The model under review builds one solid part; all positions refer to its coordinate system, in mm. A direction names the side the tool comes from. Give positions to 0.01 mm unless a question says otherwise; leave off trailing zeros. Order: outer loops, then holes, each group sorted by start corner. A loop starts at its lowest first (then second) coordinate and runs counter-clockwise, first axis right, second up. Notation, with made-up numbers: (-24, 7.5) - (31, 7.5) arc R16 cw to (31, 38.5) - close; hole circle Ø9 at (-19, 4). An arc over 180 degrees is marked (long way). Use CSV: the item, a comma, the result in double quotes. Start each with the question number.
```python
from build123d import *

# Parameters (mm, degrees)
BOSS_EXTRUDE1_DEPTH                             = 53.975
SKETCH2_W                                       = 6.858
SKETCH2_H                                       = 3.429
CUT_EXTRUDE1_DEPTH                              = 55.91468839
SKETCH4_W                                       = 6.858
SKETCH4_H                                       = 3.429
CUT_EXTRUDE2_DEPTH                              = 55.91468839
F_3_CLEARANCE_HOLE1_D                           = 2.7686
CBORE_FOR_10_BUTTON_HEAD_CAP_SCREW1_D           = 5.1054
CBORE_FOR_10_BUTTON_HEAD_CAP_SCREW1_CBORE_D     = 9.92124
CBORE_FOR_10_BUTTON_HEAD_CAP_SCREW1_CBORE_DEPTH = 3.2004
FILLET1_R                                       = 1.27
FILLET3_R                                       = 1.27
FILLET5_R                                       = 1.27


with BuildPart() as part:
    # Sketch1 → Boss-Extrude1 (new body)
    with BuildSketch(Plane.XY.offset(23.6855)):
        Polygon((3.302, 6.35), (-4.064, 6.35), (-4.064, -6.35), (3.302, -6.35), (7.874, -2.54), (7.874, 2.54), align=None)
    extrude(amount=-BOSS_EXTRUDE1_DEPTH)

    # Sketch2 → Cut-Extrude1 (cut, through all)
    with BuildSketch(Plane.XY.offset(23.6855)):
        with Locations((-0.635, 4.6355)):
            Rectangle(SKETCH2_W, SKETCH2_H)
    extrude(amount=-CUT_EXTRUDE1_DEPTH, mode=Mode.SUBTRACT)

    # Sketch4 → Cut-Extrude2 (cut, through all)
    with BuildSketch(Plane.XY.offset(23.6855)):
        with Locations((-0.635, -4.6355)):
            Rectangle(SKETCH4_W, SKETCH4_H)
    extrude(amount=-CUT_EXTRUDE2_DEPTH, mode=Mode.SUBTRACT)

    # #3 Clearance Hole1 (through all)
    with Locations(Plane.ZY.offset(4.064)):
        with Locations((12.7, 0), (-12.7, 0)):
            Hole(F_3_CLEARANCE_HOLE1_D / 2)

    # CBORE for #10 Button Head Cap Screw1 (through all)
    with Locations(Plane(origin=(7.874, 0, 0), x_dir=(0, 0, -1), z_dir=(1, 0, 0))):
        with Locations((-12.7, 0), (12.7, 0)):
            CounterBoreHole(CBORE_FOR_10_BUTTON_HEAD_CAP_SCREW1_D / 2, CBORE_FOR_10_BUTTON_HEAD_CAP_SCREW1_CBORE_D / 2, CBORE_FOR_10_BUTTON_HEAD_CAP_SCREW1_CBORE_DEPTH)

    # Fillet1
    fillet1_edges = [part.edges().sort_by_distance(p)[0] for p in [
        (7.874, -2.54, 20.323251747),
        (7.874, -2.54, -23.625251747),
        (7.874, -2.54, 0),
        (7.874, 2.54, 20.323251747),
        (7.874, 2.54, 0),
        (7.874, 2.54, -23.625251747),
    ]]
    fillet(fillet1_edges, radius=FILLET1_R)

    # Fillet3
    # the kernel refuses this fillet: 1.27 mm, written as the material it takes off along each edge
    with BuildSketch(Plane(origin=(0.862897437, -8.382585469, -30.2895), x_dir=(0, 0, 1), z_dir=(0.7682212795973759, 0.6401843996644799, 0)), Plane(origin=(7.417034188, 2.920804844, -30.2895), x_dir=(0, 0, 1), z_dir=(-0.7682212795973759, 0.6401843996644799, 0))) as fillet3_piece_1:
        with BuildLine():
            CenterArc((FILLET3_R, -FILLET3_R), FILLET3_R, 90, 90)
            Line((0, -FILLET3_R), (0, 0))
            Line((0, 0), (FILLET3_R, 0))
        make_face()
    extrude(amount=8.531574072, mode=Mode.SUBTRACT)
    with BuildSketch(Plane(origin=(6.604, -1.945163819, -30.2895), x_dir=(0.6401843996644796, -0.7682212795973762, 0), z_dir=(-0.7682212795973762, -0.6401843996644796, 0))) as fillet3_piece_2:
        with BuildLine():
            CenterArc((1.27 - FILLET3_R, FILLET3_R), FILLET3_R, 270, 90)
            Line((1.27, FILLET3_R), (1.27, 0))
            Line((1.27, 0), (1.27 - FILLET3_R, 0))
        make_face()
    revolve(axis=Axis((6.604, -1.945163819, -30.2895), (0, 0, 1)), revolution_arc=50.194428908, mode=Mode.SUBTRACT)
    with BuildSketch(Plane(origin=(6.604, 1.945163819, -30.2895), x_dir=(0.6401843996644799, 0.7682212795973757, 0), z_dir=(-0.7682212795973757, 0.6401843996644799, 0))) as fillet3_piece_3:
        with BuildLine():
            CenterArc((1.27 - FILLET3_R, -FILLET3_R), FILLET3_R, 0, 90)
            Line((1.27, -FILLET3_R), (1.27, 0))
            Line((1.27, 0), (1.27 - FILLET3_R, 0))
        make_face()
    revolve(axis=Axis((6.604, 1.945163819, -30.2895), (0, 0, -1)), revolution_arc=50.194428908, mode=Mode.SUBTRACT)
    with BuildSketch(Plane(origin=(2.794, -2.921, -30.2895), x_dir=(0, 0, 1), z_dir=(-1, 0, 0)), Plane(origin=(-7.239, 2.921, -30.2895), x_dir=(0, 0, 1), z_dir=(1, 0, 0))) as fillet3_piece_4:
        with BuildLine():
            CenterArc((FILLET3_R, FILLET3_R), FILLET3_R, 180, 90)
            Line((0, FILLET3_R), (0, 0))
            Line((0, 0), (FILLET3_R, 0))
        make_face()
    extrude(amount=10.033, mode=Mode.SUBTRACT)
    with BuildSketch(Plane(origin=(2.794, 2.921, -30.2895), x_dir=(0, 0, 1), z_dir=(0, 1, 0)), Plane(origin=(2.794, -9.525, -30.2895), x_dir=(0, 0, 1), z_dir=(0, 1, 0))) as fillet3_piece_5:
        with BuildLine():
            CenterArc((FILLET3_R, FILLET3_R), FILLET3_R, 180, 90)
            Line((0, FILLET3_R), (0, 0))
            Line((0, 0), (FILLET3_R, 0))
        make_face()
    extrude(amount=6.604, mode=Mode.SUBTRACT)
    with BuildSketch(Plane(origin=(7.874, -1.945163819, -30.2895), x_dir=(-1, 0, 0), z_dir=(0, 1, 0))) as fillet3_piece_6:
        with BuildLine():
            CenterArc((FILLET3_R, FILLET3_R), FILLET3_R, 180, 90)
            Line((0, FILLET3_R), (0, 0))
            Line((0, 0), (FILLET3_R, 0))
        make_face()
    extrude(amount=3.890327637, mode=Mode.SUBTRACT)
    with BuildSketch(Plane(origin=(2.794, -9.525, -30.2895), x_dir=(0, 0, 1), z_dir=(0, 1, 0))) as fillet3_piece_7a_section:
        with BuildLine():
            CenterArc((FILLET3_R, FILLET3_R), FILLET3_R, 180, 90)
            Line((0, FILLET3_R), (0, 0))
            Line((0, 0), (FILLET3_R, 0))
        make_face()
    fillet3_piece_7a = extrude(amount=9.779, mode=Mode.PRIVATE)
    fillet3_piece_7a = split(fillet3_piece_7a, bisect_by=Plane(origin=(3.081521795, -2.921, -30.001978205), z_dir=(0, 1, 0)), keep=Keep.TOP, mode=Mode.PRIVATE)
    with BuildSketch(Plane(origin=(5.969, -2.921, -30.2895), x_dir=(0, 0, 1), z_dir=(-1, 0, 0))) as fillet3_piece_7b_section:
        with BuildLine():
            CenterArc((FILLET3_R, FILLET3_R), FILLET3_R, 180, 90)
            Line((0, FILLET3_R), (0, 0))
            Line((0, 0), (FILLET3_R, 0))
        make_face()
    fillet3_piece_7b = extrude(amount=13.208, mode=Mode.PRIVATE)
    fillet3_piece_7b = split(fillet3_piece_7b, bisect_by=Plane(origin=(2.794, -2.633478205, -30.001978205), z_dir=(1, 0, 0)), keep=Keep.TOP, mode=Mode.PRIVATE)
    fillet3_piece_7 = fillet3_piece_7a & fillet3_piece_7b
    add(fillet3_piece_7, mode=Mode.SUBTRACT)
    with BuildSketch(Plane(origin=(2.794, -0.254, -30.2895), x_dir=(0, 0, 1), z_dir=(0, 1, 0))) as fillet3_piece_8a_section:
        with BuildLine():
            CenterArc((FILLET3_R, FILLET3_R), FILLET3_R, 180, 90)
            Line((0, FILLET3_R), (0, 0))
            Line((0, 0), (FILLET3_R, 0))
        make_face()
    fillet3_piece_8a = extrude(amount=9.779, mode=Mode.PRIVATE)
    fillet3_piece_8a = split(fillet3_piece_8a, bisect_by=Plane(origin=(3.081521795, 2.921, -30.001978205), z_dir=(0, -1, 0)), keep=Keep.TOP, mode=Mode.PRIVATE)
    with BuildSketch(Plane(origin=(-7.239, 2.921, -30.2895), x_dir=(0, 0, 1), z_dir=(1, 0, 0))) as fillet3_piece_8b_section:
        with BuildLine():
            CenterArc((FILLET3_R, FILLET3_R), FILLET3_R, 180, 90)
            Line((0, FILLET3_R), (0, 0))
            Line((0, 0), (FILLET3_R, 0))
        make_face()
    fillet3_piece_8b = extrude(amount=13.208, mode=Mode.PRIVATE)
    fillet3_piece_8b = split(fillet3_piece_8b, bisect_by=Plane(origin=(2.794, 2.633478205, -30.001978205), z_dir=(1, 0, 0)), keep=Keep.TOP, mode=Mode.PRIVATE)
    fillet3_piece_8 = fillet3_piece_8a & fillet3_piece_8b
    add(fillet3_piece_8, mode=Mode.SUBTRACT)

    # Fillet5
    # the kernel refuses this fillet: 1.27 mm, written as the material it takes off along each edge
    with BuildSketch(Plane(origin=(0.862897437, -8.382585469, 23.6855), x_dir=(-0.6401843996644799, 0.7682212795973759, 0), z_dir=(0.7682212795973759, 0.6401843996644799, 0)), Plane(origin=(7.417034188, 2.920804844, 23.6855), x_dir=(-0.6401843996644799, -0.7682212795973759, 0), z_dir=(-0.7682212795973759, 0.6401843996644799, 0))) as fillet5_piece_1:
        with BuildLine():
            CenterArc((FILLET5_R, -FILLET5_R), FILLET5_R, 90, 90)
            Line((0, -FILLET5_R), (0, 0))
            Line((0, 0), (FILLET5_R, 0))
        make_face()
    extrude(amount=8.531574072, mode=Mode.SUBTRACT)
    with BuildSketch(Plane(origin=(6.604, -1.945163819, 23.6855), x_dir=(1, 0, 0), z_dir=(0, 1, 0))) as fillet5_piece_2:
        with BuildLine():
            CenterArc((1.27 - FILLET5_R, FILLET5_R), FILLET5_R, 270, 90)
            Line((1.27, FILLET5_R), (1.27, 0))
            Line((1.27, 0), (1.27 - FILLET5_R, 0))
        make_face()
    revolve(axis=Axis((6.604, -1.945163819, 23.6855), (0, 0, -1)), revolution_arc=50.194428908, mode=Mode.SUBTRACT)
    with BuildSketch(Plane(origin=(6.604, 1.945163819, 23.6855), x_dir=(0.6401843996644799, 0.7682212795973757, 0), z_dir=(-0.7682212795973757, 0.6401843996644799, 0))) as fillet5_piece_3:
        with BuildLine():
            CenterArc((1.27 - FILLET5_R, FILLET5_R), FILLET5_R, 270, 90)
            Line((1.27, FILLET5_R), (1.27, 0))
            Line((1.27, 0), (1.27 - FILLET5_R, 0))
        make_face()
    revolve(axis=Axis((6.604, 1.945163819, 23.6855), (0, 0, -1)), revolution_arc=50.194428908, mode=Mode.SUBTRACT)
    with BuildSketch(Plane(origin=(2.794, 2.921, 23.6855), x_dir=(1, 0, 0), z_dir=(0, 1, 0)), Plane(origin=(2.794, -9.525, 23.6855), x_dir=(1, 0, 0), z_dir=(0, 1, 0))) as fillet5_piece_4:
        with BuildLine():
            CenterArc((FILLET5_R, FILLET5_R), FILLET5_R, 180, 90)
            Line((0, FILLET5_R), (0, 0))
            Line((0, 0), (FILLET5_R, 0))
        make_face()
    extrude(amount=6.604, mode=Mode.SUBTRACT)
    with BuildSketch(Plane(origin=(-7.239, 2.921, 23.6855), x_dir=(0, -1, 0), z_dir=(1, 0, 0)), Plane(origin=(2.794, -2.921, 23.6855), x_dir=(0, 1, 0), z_dir=(-1, 0, 0))) as fillet5_piece_5:
        with BuildLine():
            CenterArc((FILLET5_R, FILLET5_R), FILLET5_R, 180, 90)
            Line((0, FILLET5_R), (0, 0))
            Line((0, 0), (FILLET5_R, 0))
        make_face()
    extrude(amount=10.033, mode=Mode.SUBTRACT)
    with BuildSketch(Plane(origin=(7.874, -1.945163819, 23.6855), x_dir=(-1, 0, 0), z_dir=(0, 1, 0))) as fillet5_piece_6:
        with BuildLine():
            CenterArc((FILLET5_R, -FILLET5_R), FILLET5_R, 90, 90)
            Line((0, -FILLET5_R), (0, 0))
            Line((0, 0), (FILLET5_R, 0))
        make_face()
    extrude(amount=3.890327637, mode=Mode.SUBTRACT)
    with BuildSketch(Plane(origin=(2.794, -0.254, 23.6855), x_dir=(1, 0, 0), z_dir=(0, 1, 0))) as fillet5_piece_7a_section:
        with BuildLine():
            CenterArc((FILLET5_R, FILLET5_R), FILLET5_R, 180, 90)
            Line((0, FILLET5_R), (0, 0))
            Line((0, 0), (FILLET5_R, 0))
        make_face()
    fillet5_piece_7a = extrude(amount=9.779, mode=Mode.PRIVATE)
    fillet5_piece_7a = split(fillet5_piece_7a, bisect_by=Plane(origin=(3.081521795, 2.921, 23.397978205), z_dir=(0, -1, 0)), keep=Keep.TOP, mode=Mode.PRIVATE)
    with BuildSketch(Plane(origin=(-7.239, 2.921, 23.6855), x_dir=(0, -1, 0), z_dir=(1, 0, 0))) as fillet5_piece_7b_section:
        with BuildLine():
            CenterArc((FILLET5_R, FILLET5_R), FILLET5_R, 180, 90)
            Line((0, FILLET5_R), (0, 0))
            Line((0, 0), (FILLET5_R, 0))
        make_face()
    fillet5_piece_7b = extrude(amount=13.208, mode=Mode.PRIVATE)
    fillet5_piece_7b = split(fillet5_piece_7b, bisect_by=Plane(origin=(2.794, 2.633478205, 23.397978205), z_dir=(1, 0, 0)), keep=Keep.TOP, mode=Mode.PRIVATE)
    fillet5_piece_7 = fillet5_piece_7a & fillet5_piece_7b
    add(fillet5_piece_7, mode=Mode.SUBTRACT)
    with BuildSketch(Plane(origin=(2.794, -9.525, 23.6855), x_dir=(1, 0, 0), z_dir=(0, 1, 0))) as fillet5_piece_8a_section:
        with BuildLine():
            CenterArc((FILLET5_R, FILLET5_R), FILLET5_R, 180, 90)
            Line((0, FILLET5_R), (0, 0))
            Line((0, 0), (FILLET5_R, 0))
        make_face()
    fillet5_piece_8a = extrude(amount=9.779, mode=Mode.PRIVATE)
    fillet5_piece_8a = split(fillet5_piece_8a, bisect_by=Plane(origin=(3.081521795, -2.921, 23.397978205), z_dir=(0, 1, 0)), keep=Keep.TOP, mode=Mode.PRIVATE)
    with BuildSketch(Plane(origin=(5.969, -2.921, 23.6855), x_dir=(0, 1, 0), z_dir=(-1, 0, 0))) as fillet5_piece_8b_section:
        with BuildLine():
            CenterArc((FILLET5_R, FILLET5_R), FILLET5_R, 180, 90)
            Line((0, FILLET5_R), (0, 0))
            Line((0, 0), (FILLET5_R, 0))
        make_face()
    fillet5_piece_8b = extrude(amount=13.208, mode=Mode.PRIVATE)
    fillet5_piece_8b = split(fillet5_piece_8b, bisect_by=Plane(origin=(2.794, -2.633478205, 23.397978205), z_dir=(1, 0, 0)), keep=Keep.TOP, mode=Mode.PRIVATE)
    fillet5_piece_8 = fillet5_piece_8a & fillet5_piece_8b
    add(fillet5_piece_8, mode=Mode.SUBTRACT)


solid = part.part
```
1. To check wall thickness, follow L1, parallel to Z at x = 6.65, y = 0; L2, parallel to Z at x = 6, y = 2; L3, parallel to Y at x = -0.25, z = -24. State the ranges of each line that lie inside material, in increasing order. Write a range as [from, to].
2. Mouldability with a two-part tool opening along Y and no side actions: class faces 1 (the face through (4.994, -4.443, 23.323)), 2 (the face through (2.794, -5, -3)), 3 (the face through (0.244, 0.767, 15.135)) as pulls with the +Y half, pulls with the -Y half, needs draft (parallel to the pull), parting line crosses it, or undercut.
3. Consider section B-B (z = -12.7). Give the boundary of the cut face in (x, y).
4. Consider section D-D (z = -20.5). Give the boundary of the cut face in (x, y).
5. Tool access review of faces 4 (the face through (4.674, 1, -10)), 5 (the face through (-1, -2.921, -4)), 6 (the face through (-0.057, 2.539, -29.927)), 7 (the face through (0.057, -2.539, -29.927)): name each direction out of +Z, -Z, +X, -X, +Y, -Y from which nothing blocks a thin tool from reaching the whole face with its end or side.
6. Clearance check with flat-ended pins moving along their axes: pin 1 (3 mm diameter, centred on y = 0.5, z = -14, fed in from +X); pin 2 (1 mm diameter, centred on y = 5.5, z = -15, fed in from -X); pin 3 (3 mm diameter, centred on x = 0, z = -18, fed in from +Y). State where each tip first meets the part, or that it passes through.
7. Consider section C-C (x = -0.5). Give the boundary of the cut face in (y, z).
8. Consider section A-A (y = 0). Give the boundary of the cut face in (x, z).
Answers follow:
1,L1,"z = [-30.29, -17.66], [-7.74, 7.74], [17.66, 23.68]"
1,L2,"z = [-30.29, -17.24], [-8.16, 8.16], [17.24, 23.69]"
1,L3,"y = [-2.92, 2.92]"
2,face 1,"pulls with the -Y half"
2,face 2,"needs draft"
2,face 3,"undercut"
3,outline,"(-4.06, -2.92) - (2.79, -2.92) - (2.79, -6.35) - (3.3, -6.35) - (4.97, -4.96) - (4.67, -4.96) - (4.67, -2.55) - (-4.06, -2.55) - close; (-4.06, 2.55) - (4.67, 2.55) - (4.67, 4.96) - (4.97, 4.96) - (3.3, 6.35) - (2.79, 6.35) - (2.79, 2.92) - (-4.06, 2.92) - close"
4,outline,"(-4.06, -2.92) - (2.79, -2.92) - (2.79, -6.35) - (3.3, -6.35) - (7.42, -2.92) arc R1.27 ccw to (7.87, -1.95) - (7.87, 1.95) arc R1.27 ccw to (7.42, 2.92) - (3.3, 6.35) - (2.79, 6.35) - (2.79, 2.92) - (-4.06, 2.92) - close"
5,face 4,"+X"
5,face 5,"+Z, -Z, -X, -Y"
5,face 6,"-Z, -X, +Y"
5,face 7,"-Z, -X, -Y"
6,pin 1,"stops at x = 4.67"
6,pin 2,"stops at x = 2.79"
6,pin 3,"stops at y = 2.92"
7,outline,"(-2.92, -29.02) arc R1.27 ccw to (-1.65, -30.29) - (1.65, -30.29) arc R1.27 ccw to (2.92, -29.02) - (2.92, 22.42) arc R1.27 ccw to (1.65, 23.69) - (-1.65, 23.69) arc R1.27 ccw to (-2.92, 22.42) - close; hole circle Ø5.11 at (0, -12.7); hole circle Ø5.11 at (0, 12.7)"
8,outline,"(-4.06, -30.29) - (6.6, -30.29) arc R1.27 ccw to (7.87, -29.02) - (7.87, -17.66) - (4.67, -17.66) - (4.67, -15.25) - (-4.06, -15.25) - close; (-4.06, -10.15) - (4.67, -10.15) - (4.67, -7.74) - (7.87, -7.74) - (7.87, 7.74) - (4.67, 7.74) - (4.67, 10.15) - (-4.06, 10.15) - close; (-4.06, 15.25) - (4.67, 15.25) - (4.67, 17.66) - (7.87, 17.66) - (7.87, 22.42) arc R1.27 ccw to (6.6, 23.69) - (-4.06, 23.69) - close"
